```python
from build123d import *

# Parameters (mm, degrees)
EXTRUDE_1_DEPTH           = 400
HOLE_WIZARD_1_D           = 6
HOLE_WIZARD_1_CBORE_D     = 9.5
HOLE_WIZARD_1_CBORE_DEPTH = 8.5
PATTERN_LINEAR_1_COUNT    = 7
PATTERN_LINEAR_1_PITCH    = 60


with BuildPart() as part:
    # 草图1 → 凸台-拉伸1 (new body)
    with BuildSketch(Plane.XY):
        with BuildLine():
            Line((0.146446607, 14.877167225), (0.33665166, 15.067372278))
            ThreePointArc((0.33665166, 15.067372278), (0.456581276, 15.155881832), (0.597272425, 15.205106231))
            ThreePointArc((0.597272425, 15.205106231), (1.655392341, 15.764307144), (2.214593278, 16.822427055))
            ThreePointArc((2.214593278, 16.822427055), (2.263817599, 16.96311829), (2.3523274, 17.083047759))
            Line((2.3523274, 17.083047759), (2.769279462, 17.499999821))
            Line((2.769279462, 17.499999821), (17.230720684, 17.499999821))
            Line((17.230720684, 17.499999821), (17.647672747, 17.083047759))
            ThreePointArc((17.647672747, 17.083047759), (17.736182286, 16.963118168), (17.785406689, 16.822427051))
            ThreePointArc((17.785406689, 16.822427051), (18.344607694, 15.764307233), (19.402727615, 15.205106406))
            ThreePointArc((19.402727615, 15.205106406), (19.54341887, 15.155882087), (19.663348354, 15.067372278))
            Line((19.663348354, 15.067372278), (19.853553407, 14.877167225))
            ThreePointArc((19.853553407, 14.877167225), (19.961939783, 14.714955551), (20.000000017, 14.523613835))
            Line((20.000000017, 14.523613835), (20.000000017, 13.466386174))
            ThreePointArc((20.000000017, 13.466386174), (19.961939783, 13.275044458), (19.853553407, 13.112832784))
            Line((19.853553407, 13.112832784), (19.675343411, 12.934622787))
            ThreePointArc((19.675343411, 12.934622787), (19.554347233, 12.845550893), (19.412352183, 12.796446074))
            ThreePointArc((19.412352183, 12.796446074), (18.344607801, 12.23544862), (17.783610347, 11.167704238))
            ThreePointArc((17.783610347, 11.167704238), (17.734505529, 11.025709189), (17.645433635, 10.904713011))
            Line((17.645433635, 10.904713011), (16.892893236, 10.152172612))
            ThreePointArc((16.892893236, 10.152172612), (16.676120484, 9.827749263), (16.600000023, 9.44506583))
            Line((16.600000023, 9.44506583), (16.600000023, 7.884934177))
            ThreePointArc((16.600000023, 7.884934177), (16.67612049, 7.502250748), (16.892893231, 7.177827393))
            Line((16.892893231, 7.177827393), (19.707106793, 4.363613831))
            ThreePointArc((19.707106793, 4.363613831), (19.923879539, 4.039190479), (20.000000006, 3.656507049))
            Line((20.000000006, 3.656507049), (20.000000006, 1))
            Line((20.000000006, 1), (19.000000006, 0))
            Line((19.000000006, 0), (1.000000006, 0))
            Line((1.000000006, 0), (6e-09, 1))
            Line((6e-09, 1), (6e-09, 3.656507049))
            ThreePointArc((6e-09, 3.656507049), (0.076120462, 4.039190482), (0.292893214, 4.363613832))
            Line((0.292893214, 4.363613832), (3.107106776, 7.177827394))
            ThreePointArc((3.107106776, 7.177827394), (3.323879528, 7.502250744), (3.399999989, 7.884934177))
            Line((3.399999989, 7.884934177), (3.399999989, 9.44506583))
            ThreePointArc((3.399999989, 9.44506583), (3.323879522, 9.827749259), (3.107106778, 10.152172612))
            Line((3.107106778, 10.152172612), (2.35456638, 10.904713011))
            ThreePointArc((2.35456638, 10.904713011), (2.265494485, 11.025709189), (2.216389667, 11.167704238))
            ThreePointArc((2.216389667, 11.167704238), (1.655392213, 12.235448621), (0.587647831, 12.796446074))
            ThreePointArc((0.587647831, 12.796446074), (0.445652781, 12.845550893), (0.324656604, 12.934622787))
            Line((0.324656604, 12.934622787), (0.146446607, 13.112832784))
            ThreePointArc((0.146446607, 13.112832784), (0.038060231, 13.275044458), (-3e-09, 13.466386175))
            Line((-3e-09, 13.466386175), (-3e-09, 14.523613835))
            ThreePointArc((-3e-09, 14.523613835), (0.038060231, 14.714955551), (0.146446607, 14.877167225))
        make_face()
    extrude(amount=-EXTRUDE_1_DEPTH)

    # 打孔尺寸根据内六角圆柱头螺钉的类型1 (through all)
    with Locations(Plane(origin=(0, 17.499999821, 0), x_dir=(1, 0, 0), z_dir=(0, 1, 0))):
        with Locations((10.000000073, 20)):
            hole_wizard_1 = CounterBoreHole(HOLE_WIZARD_1_D / 2, HOLE_WIZARD_1_CBORE_D / 2, HOLE_WIZARD_1_CBORE_DEPTH)

    # 阵列(线性)1: 打孔尺寸根据内六角圆柱头螺钉的类型1 ×7
    with Locations(*[(0, 0, -i * PATTERN_LINEAR_1_PITCH) for i in range(1, PATTERN_LINEAR_1_COUNT)]):
        add(hole_wizard_1, mode=Mode.SUBTRACT)


solid = part.part
```
Could you check a few things on this model? Use its own coordinates, in mm. A direction names the side the tool comes from. Round coordinates to 2 decimals unless told otherwise and drop trailing zeros. Answer in a Markdown table with one row per item. Add a question column.
Q1. If I drill on line 1 (X direction, y = 14.75, z = -320); line 2 (X direction, y = 5, z = -380); line 3 (Y direction, x = 2, z = -196.5), over which ranges is the centre line in solid material (lowest first)? Write a range as from..to.
Q2. Will these pins go through, and if not, where does the flat tip stop? pin 1 Ø5 at (x, z) = (8, -320) entering from +Y; pin 2 Ø0.8 at (y, z) = (9, -211.5) entering from +X; pin 3 Ø2 at (y, z) = (5, -318) entering from +X.
Q3. On a 3-axis mill with a long thin cutter (end or side, diameter ignored), from which of +Z, -Z, +X, -X, +Y, -Y can I reach the whole of each face in a straight line? I mean faces 4 (the flat face through (10, 9, -400)), 5 (the flat face through (13, 9, -79)). Say none if no direction works.
Q4. If we mould it in two halves opening along Z, with no side actions, what happens to faces 1 (the flat face through (10, 9, 0)), 2 (the flat face through (12, 0, -197)), 3 (the flat face through (11, 9, -197))? For each: +Z half, -Z half, draft (parallel to the pull), parting line (faces both ways), or undercut.
Values:
| question | item | result |
|---|---|---|
| 1 | line 1 | 0.05..5.25, 14.75..19.95 |
| 1 | line 2 | 0.93..7, 13..19.07 |
| 1 | line 3 | 0..6.07, 11.78..16.22 |
| 2 | pin 1 | y = 9 |
| 2 | pin 2 | x = 16.6 |
| 2 | pin 3 | x = 19.94 |
| 3 | face 4 | -Z, +X, -X, +Y, -Y |
| 3 | face 5 | +Y |
| 4 | face 1 | +Z half |
| 4 | face 2 | draft |
| 4 | face 3 | undercut |
